The listing builds one solid part. Answer for the finished solid, in the listing's coordinates (mm). A direction names the side the tool comes from. Round coordinates to 2 decimals unless told otherwise and drop trailing zeros. Loops run counter-clockwise (first coordinate to the right, second up) from the corner with the lowest first, then second, coordinate; pieces in that order, holes last. Notation, with made-up numbers: M -2,52 L 35,52 A30 cw 35,84 Z; hole C 12,71 d4. An arc over 180 degrees is marked long. Answer as a JSON object with one key per item and string values.
```python
from build123d import *

# Parameters (mm, degrees)
CYLINDER092_R     = 3.15
CYLINDER092_DEPTH = 10
CYLINDER096_R     = 0.6
CYLINDER096_DEPTH = 20
BOX047_W          = 12
BOX047_H          = 23
BOX047_DEPTH      = 10
CHAMFER006_SIZE   = 3
CHAMFER007_SIZE   = 1
CYLINDER093_R     = 3.15
CYLINDER093_DEPTH = 10
PAD008_DEPTH      = 10
CHAMFER011_SIZE2  = 50
CHAMFER011_SIZE   = 7
FILLET063_R       = 1
FILLET064_R       = 1
FILLET062_R       = 4
CYLINDER120_R     = 1.4
CYLINDER120_DEPTH = 2.5
FILLET065_R       = 4


with BuildPart() as zylinder092:
    # Cylinder092 → Cylinder092 (new body)
    with BuildSketch(Plane(origin=(-52.5, 10, -1), x_dir=(1, 0, 0), z_dir=(0, 0, 1))):
        Circle(CYLINDER092_R)
    extrude(amount=CYLINDER092_DEPTH)


with BuildPart() as zylinder096:
    # Cylinder096 → Cylinder096 (new body)
    with BuildSketch(Plane(origin=(-52.5, 23, -38.5), x_dir=(1, 0, 0), z_dir=(0, 0, 1))):
        Circle(CYLINDER096_R)
    extrude(amount=CYLINDER096_DEPTH)


with BuildPart() as chamfer007:
    # Box047 → Box047 (new body)
    with BuildSketch(Plane(origin=(-58.5, 3.5, -2.5), x_dir=(1, 0, 0), z_dir=(0, 0, 1))):
        with Locations((6, 11.5)):
            Rectangle(BOX047_W, BOX047_H)
    extrude(amount=BOX047_DEPTH)

    # Chamfer006
    chamfer006_edges = [chamfer007.edges().sort_by_distance(p)[0] for p in [
        (-52.5, 26.5, 7.5),
    ]]
    chamfer(chamfer006_edges, length=CHAMFER006_SIZE)

    # Chamfer007
    chamfer007_edges = [chamfer007.edges().sort_by_distance(p)[0] for p in [
        (-52.5, 26.5, 4.5),
    ]]
    chamfer(chamfer007_edges, length=CHAMFER007_SIZE)


with BuildPart() as fusion072:
    # Cylinder093 → Cylinder093 (new body)
    with BuildSketch(Plane(origin=(-52.5, 10, -31.5), x_dir=(1, 0, 0), z_dir=(0, 0, 1))):
        Circle(CYLINDER093_R)
    extrude(amount=CYLINDER093_DEPTH)

    # Fusion072: union Zylinder092, Zylinder096, Chamfer007
    add(zylinder092.part)
    add(zylinder096.part)
    add(chamfer007.part)


with BuildPart() as fillet062:
    # Sketch008 → Pad008 (new body)
    with BuildSketch(Plane.YZ):
        with BuildLine():
            Line((16, 4), (4, 4))
            Line((4, 4), (4, 10))
            Line((4, 10), (21, 10))
            add(Edge.make_bspline(
                [(21, 10), (33, 12), (40, 18)],
                knots=[0, 0, 0, 1, 1, 1], degree=2))
            add(Edge.make_bspline(
                [(40, 18), (42, 12), (49, 7)],
                knots=[0, 0, 0, 1, 1, 1], degree=2))
            add(Edge.make_bspline(
                [(49, 7), (50, -43)],
                knots=[0, 0, 1, 1], degree=1))
            Line((50, -43), (48, -43))
            add(Edge.make_bspline(
                [(48, -43), (48, 10), (38, 10)],
                knots=[0, 0, 0, 1, 1, 1], degree=2))
            add(Edge.make_bspline(
                [(28, -33), (31.54521, 5.416211), (38, 10)],
                knots=[0, 0, 0, 1, 1, 1], degree=2))
            Line((28, -33), (5, -33))
            Line((5, -33), (5, -29))
            Line((5, -29), (18, -29))
            add(Edge.make_bspline(
                [(21, 6), (25.7922, 6), (28.2733, -3.63721), (27.206068, -18.457365), (25.411083, -30.376215), (22.292137, -30), (18, -29)],
                knots=[0, 0, 0, 0, 0.25, 0.5, 0.75, 1, 1, 1, 1], degree=3))
            Line((21, 6), (16, 4))
        make_face()
    extrude(amount=PAD008_DEPTH)

    # Chamfer011
    chamfer011_edges = [fillet062.edges().sort_by_distance(p)[0] for p in [
        (0, 49, -43),
    ]]
    chamfer011_side = fillet062.faces().sort_by_distance((5, 49, -43))[0]
    chamfer(chamfer011_edges, length=CHAMFER011_SIZE, length2=CHAMFER011_SIZE2, reference=chamfer011_side)


with BuildPart() as fillet062_1:
    # Chamfer011 placement: moved
    add(fillet062.part.moved(Location((11.5, 0, 0))))

    # Fillet063
    fillet063_edges = [fillet062_1.edges().sort_by_distance(p)[0] for p in [
        (16.5, 49, 7),
    ]]
    fillet(fillet063_edges, radius=FILLET063_R)

    # Fillet064
    fillet064_edges = [fillet062_1.edges().sort_by_distance(p)[0] for p in [
        (16.5, 28, -33),
    ]]
    fillet(fillet064_edges, radius=FILLET064_R)

    # Fillet062
    fillet062_edges = [fillet062_1.edges().sort_by_distance(p)[0] for p in [
        (21.5, 4, 7),
        (11.5, 4, 7),
    ]]
    fillet(fillet062_edges, radius=FILLET062_R)


with BuildPart() as fillet065:
    # Cylinder120 → Cylinder120 (new body)
    with BuildSketch(Plane(origin=(16.5, 23, -35.5), x_dir=(1, 0, 0), z_dir=(0, 0, 1))):
        Circle(CYLINDER120_R)
    extrude(amount=CYLINDER120_DEPTH)

    # Fusion080: union Fillet062
    add(fillet062_1.part)


with BuildPart() as fillet065_1:
    # Fusion080 placement: moved
    add(fillet065.part.moved(Location((-69, 0, 0))))

    # Cut060: cut Fusion072
    add(fusion072.part, mode=Mode.SUBTRACT)

    # Fillet065
    fillet065_edges = [fillet065_1.edges().sort_by_distance(p)[0] for p in [
        (-47.5, 5, -31),
        (-57.5, 5, -31),
    ]]
    fillet(fillet065_edges, radius=FILLET065_R)


solid = fillet065_1.part
```
Item 1: Which of the six approach directions +Z, -Z, +X, -X, +Y, -Y give full straight-line access (tool end or side, diameter ignored) to faces 5 (the face through (-48.641, 6.203, -30.972)), 6 (the face through (-52.57, 26.14, 4.37)), 7 (the face through (-53, 10, -31.5))?
Values follow:
{"face 5": "-Z, +X, -Y", "face 6": "+X, -X, -Y", "face 7": "none"}
Item 2: The part is cut by section A-A (y = 14.5). Give the vertices of the cut face in (x, z).
Values follow:
{"outline": "M -57.5,-33 L -47.5,-33 L -47.5,-29 L -57.5,-29 Z; M -57.5,7.5 L -47.5,7.5 L -47.5,10 L -57.5,10 Z"}
Item 3: Flat-ended cylindrical pins translate along their axes: P1, Ø3, axis at x = -52.5, y = 23, coming from the -Z side; P2, Ø5, axis at x = -50, y = 19.5, coming from the -Z side; P3, Ø3, axis at x = -51, y = 10.5, coming from the +Z side; P4, Ø3, axis at y = 23.5, z = 0.5, coming from the +X side. Find the tip coordinate at first contact, or state that the pin passes through.
Values follow:
{"P1": "z = -35.5", "P2": "z = -33", "P3": "z = 10", "P4": "through"}
Item 4: Determine the mould class of faces 1 (the face through (-53, 12, 10)), 2 (the face through (-53, 22, -35.5)), 3 (the face through (-53, 10, 9)), 4 (the face through (-56.297, 5.141, 8.768)) for opening direction Z: released by +Z, released by -Z, zero draft, split by the parting line, or undercut.
Values follow:
{"face 1": "released by +Z", "face 2": "released by -Z", "face 3": "undercut", "face 4": "zero draft"}
Item 5: Straight lines are drawn through the part: line 1 (Z direction, x = -53, y = 15.5); line 2 (Y direction, x = -52.5, z = 8); line 3 (Y direction, x = -52.5, z = 8.5). For each, find the intervals that lie inside material, in ascending order.
Values follow:
{"line 1": "-33 to -29, 7.5 to 10", "line 2": "4 to 6.85, 13.15 to 36.22, 41.51 to 47.66", "line 3": "4 to 6.85, 13.15 to 36.56, 41.08 to 47.04"}
